For this review, take the finished solid that the model builds, in its own axes (mm). Face numbers are marked on the shaded views. Give positions to 0.01 mm unless a question says otherwise; leave off trailing zeros. Loops run counter-clockwise (first coordinate to the right, second up) from the corner with the lowest first, then second, coordinate; pieces in that order, holes last. Notation, with made-up numbers: (0, 37.25) - (12, 37.25) arc R30 ccw to (12, 66.25) - close; hole circle Ø4 at (3.5, 23.25). An arc over 180 degrees is marked (long way). Answer in a Markdown table with one row per item.
```python
from build123d import *

# Parameters (mm, degrees)
F0_R     = 34.925
F1_DEPTH = 9.525
F0_R_2   = 38.1
F2_DEPTH = 123.825


# Not quite as in the source:
# - a fillet or chamfer that OpenCascade refuses, or shapes differently, is made with other operations: its cross-section is extruded or revolved along the edge and cut away or added


with BuildPart() as f1:
    # F0 (on Front) → F1 (new body)
    with BuildSketch(Plane.XZ):
        Circle(F0_R)
    extrude(amount=F1_DEPTH)

    # F0 (on Front) → F2 (join)
    with BuildSketch(Plane.XZ):
        Circle(F0_R_2)
        Circle(F0_R, mode=Mode.SUBTRACT)
    extrude(amount=F2_DEPTH)

    # F3: fillet of radius 6.35 on 1 edges, made by hand

    # F3_s1 → F3_t2 (revolve, cut)
    with BuildSketch(Plane.XY):
        with BuildLine():
            ThreePointArc((38.1, -118.325738686), (37.249261314, -121.500738686), (34.925, -123.825))
            Line((34.925, -123.825), (38.1, -123.825))
            Line((38.1, -123.825), (38.1, -118.325738686))
        make_face()
    revolve(axis=Axis((0, -123.825, 0), (0, -1, 0)), mode=Mode.SUBTRACT)


solid = f1.part
```
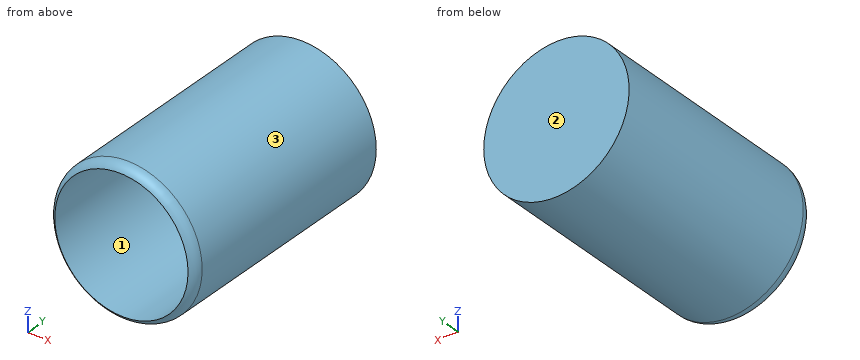
1. Mouldability with a two-part tool opening along Z and no side actions: class the marked faces 1, 2 and 3 as released by +Z, released by -Z, zero draft, split by the parting line, or undercut.
Values:
| item | result |
|---|---|
| face 1 | undercut |
| face 2 | zero draft |
| face 3 | split by the parting line |
2. Clearance check with flat-ended pins moving along their axes: pin 1 (1.5 mm diameter, centred on x = 26.5, y = -75, fed in from +Z); pin 2 (2 mm diameter, centred on x = 4, y = -25, fed in from -Z); pin 3 (12 mm diameter, centred on x = 30, y = -47.5, fed in from +Z). State where each tip first meets the part, or that it passes through.
Values:
| item | result |
|---|---|
| pin 1 | stops at z = 28.08 |
| pin 2 | stops at z = -37.98 |
| pin 3 | stops at z = 29.59 |
3. We need section B-B, the plane y = -76. Give the boundary of the cut face in (x, z) (3 decimals), and give its area (3 significant figures).
Values:
| item | result |
|---|---|
| outline | circle Ø76.2 at (0, 0); hole circle Ø69.85 at (0, 0) |
| area | 728 mm^2 |
4. We need section C-C, the plane x = 0. Give the boundary of the cut face in (y, z) (3 decimals).
Values:
| item | result |
|---|---|
| outline | (-123.825, -34.925) arc R6.35 ccw to (-118.326, -38.1) - (0, -38.1) - (0, 38.1) - (-118.326, 38.1) arc R6.35 ccw to (-123.825, 34.925) - (-9.525, 34.925) - (-9.525, -34.925) - close |
5. We need section A-A, the plane z = 0. Give the boundary of the cut face in (x, y) (3 decimals), and give its area (3 significant figures).
Values:
| item | result |
|---|---|
| outline | (-38.1, -118.326) arc R6.35 ccw to (-34.925, -123.825) - (-34.925, -9.525) - (34.925, -9.525) - (34.925, -123.825) arc R6.35 ccw to (38.1, -118.326) - (38.1, 0) - (-38.1, 0) - close |
| area | 1,440 mm^2 |
6. Wall thickness on line 1 (Z direction, x = 0, y = -71) (3 decimals); line 2 (Y direction, x = -10, z = -30) (3 decimals); line 3 (Z direction, x = 18, y = -32.5): over which ranges is each line inside the solid? List them lowest first. Write a range as [from, to].
Values:
| item | result |
|---|---|
| line 1 | z = [-38.1, -34.925], [34.925, 38.1] |
| line 2 | y = [-9.525, 0] |
| line 3 | z = [-33.58, -29.93], [29.93, 33.58] |
